```python
from build123d import *

# Parameters (mm, degrees)
SKETCH1_W           = 650
SKETCH1_H           = 300
SKETCH1_W_2         = 175
SKETCH1_H_2         = 150
BOSS_EXTRUDE1_DEPTH = 75
SKETCH2_W           = 240
SKETCH2_H           = 185
CUT_EXTRUDE1_DEPTH  = 125
CUT_EXTRUDE2_DEPTH  = 100
SKETCH4_W           = 30
SKETCH4_H           = 500
BOSS_EXTRUDE2_DEPTH = 30


with BuildPart() as part:
    # Sketch1 → Boss-Extrude1 (new, symmetric)
    with BuildSketch(Plane(origin=(0, 0, 0), x_dir=(1, 0, 0), z_dir=(0, 1, 0))):
        Rectangle(SKETCH1_W, SKETCH1_H)
        with Locations((-412.5, 0)):
            Rectangle(SKETCH1_W_2, SKETCH1_H)
        with Locations((0, -225)):
            Rectangle(SKETCH1_W, SKETCH1_H_2)
        with Locations((412.5, 0)):
            Rectangle(SKETCH1_W_2, SKETCH1_H)
        with Locations((0, 225)):
            Rectangle(SKETCH1_W, SKETCH1_H_2)
    extrude(amount=BOSS_EXTRUDE1_DEPTH, both=True)

    # Sketch2 → Cut-Extrude1 (cut)
    with BuildSketch(Plane(origin=(0, 75, 0), x_dir=(1, 0, 0), z_dir=(0, 1, 0))):
        Rectangle(SKETCH2_W, SKETCH2_H)
    extrude(amount=-CUT_EXTRUDE1_DEPTH, mode=Mode.SUBTRACT)

    # Sketch3 → Cut-Extrude2 (cut)
    with BuildSketch(Plane(origin=(0, 75, 0), x_dir=(1, 0, 0), z_dir=(0, 1, 0))):
        Polygon((-450, 100), (-275, 100), (-275, 250), (275, 250), (275, 100), (450, 100), (450, -100), (275, -100), (275, -250), (-275, -250), (-275, -100), (-450, -100), align=None)
    extrude(amount=-CUT_EXTRUDE2_DEPTH, mode=Mode.SUBTRACT)

    # Sketch4 → Boss-Extrude2 (add)
    with BuildSketch(Plane(origin=(0, 75, 0), x_dir=(1, 0, 0), z_dir=(0, 1, 0))):
        with Locations((-135, 0)):
            Rectangle(SKETCH4_W, SKETCH4_H)
        with Locations((135, 0)):
            Rectangle(SKETCH4_W, SKETCH4_H)
    extrude(amount=-BOSS_EXTRUDE2_DEPTH)


solid = part.part
```
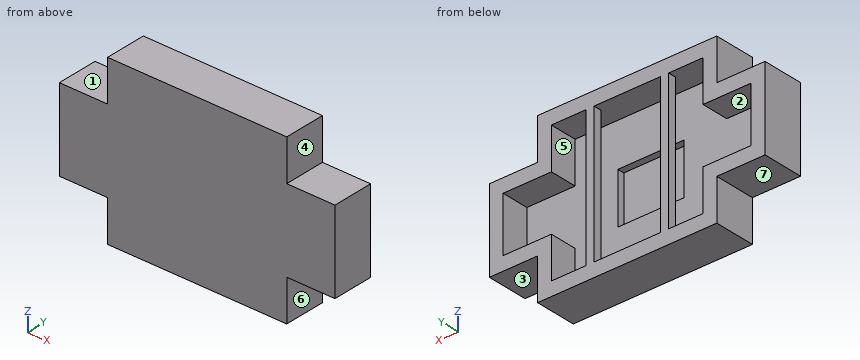
The listing builds one solid part. Answer for the finished solid, in the listing's coordinates (mm). Face numbers are marked on the shaded views. A direction names the side the tool comes from. Give positions to 0.01 mm unless a question says otherwise; leave off trailing zeros. Write each loop counter-clockwise with the first axis right and the second up, starting at its lowest first coordinate (ties: lowest second). Pieces come first, ordered by that corner, then holes. Notation, with made-up numbers: (68.25, 59.5) -> (121.25, 59.5) arc R26 ccw to (121.25, 87.5) -> close; hole circle Ø6 at (40, 51). An arc over 180 degrees is marked (long way). Use one line per item in the form item = value.
1) For a pull along Z with two mould halves and no side action, classify the marked faces 5, 6 and 7 as +Z half, -Z half, draft (parallel to the pull), parting line (faces both ways), or undercut.
Result:
face_5 = undercut
face_6 = draft
face_7 = -Z half
2) Straight lines are drawn through the part: probe 1 along X at (y, z) = (57, 0); probe 2 along Z at (x, y) = (-203, 2); probe 3 along Z at (x, y) = (338.5, -14.5). For each, find the intervals that lie inside material, in ascending order.
Result:
probe_1 = -500 to -450, -150 to -120, 120 to 150, 450 to 500
probe_2 = -300 to -250, 250 to 300
probe_3 = -150 to -100, 100 to 150
3) Section A-A on z = -111.5 is taken. Write down the section's boundary in (x, y), plus the area to 3 significant figures.
Result:
outline = (-500, -75) -> (500, -75) -> (500, 75) -> (275, 75) -> (275, -25) -> (-275, -25) -> (-275, 75) -> (-500, 75) -> close; (-150, 45) -> (-120, 45) -> (-120, 75) -> (-150, 75) -> close; (120, 45) -> (150, 45) -> (150, 75) -> (120, 75) -> close
area = 96,800 mm²
4) Section B-B on x = 165 is taken. Write down the section's boundary in (y, z).
Result:
outline = (-75, -300) -> (75, -300) -> (75, -250) -> (-25, -250) -> (-25, 250) -> (75, 250) -> (75, 300) -> (-75, 300) -> close
5) Section D-D on z = 200 is taken. Write down the section's boundary in (x, y), plus the area to 3 significant figures.
Result:
outline = (-325, -75) -> (325, -75) -> (325, 75) -> (275, 75) -> (275, -25) -> (-275, -25) -> (-275, 75) -> (-325, 75) -> close; (-150, 45) -> (-120, 45) -> (-120, 75) -> (-150, 75) -> close; (120, 45) -> (150, 45) -> (150, 75) -> (120, 75) -> close
area = 44,300 mm²
6) Section C-C on y = -10.5 is taken. Write down the section's boundary in (x, z).
Result:
outline = (-500, -150) -> (-325, -150) -> (-325, -300) -> (325, -300) -> (325, -150) -> (500, -150) -> (500, 150) -> (325, 150) -> (325, 300) -> (-325, 300) -> (-325, 150) -> (-500, 150) -> close; hole (-450, -100) -> (-275, -100) -> (-275, -250) -> (275, -250) -> (275, -100) -> (450, -100) -> (450, 100) -> (275, 100) -> (275, 250) -> (-275, 250) -> (-275, 100) -> (-450, 100) -> close
7) Each of these flat-tipped pins is pushed along its axis until it touches: P1, Ø10, axis at y = -52, z = 204, coming from the -X side; P2, Ø1, axis at x = 181.5, z = 25, coming from the +Y side. Where does it stop, or does it pass through?
Result:
P1 = -325
P2 = -25
8) A tool of negligible diameter and unlimited length cuts with its end or side. For the marked faces 1, 2, 3 and 4, from which of +Z, -Z, +X, -X, +Y, -Y can it reach the whole face along a straight path? Write none if from no direction.
Result:
face_1 = +Z, -X, +Y, -Y
face_2 = +Y
face_3 = -Z, +X, +Y, -Y
face_4 = +Z, +X, +Y, -Y
